```python
from build123d import *

# Parameters (mm, degrees)
BOSS_EXTRUDE1_DEPTH = 1.5
FILLET1_R           = 1.5875
SKETCH2_W           = 3
SKETCH2_H           = 6.35
BOSS_EXTRUDE2_DEPTH = 3
FILLET2_R           = 0.79375


with BuildPart() as part:
    # Sketch1 → Boss-Extrude1 (new, symmetric)
    with BuildSketch(Plane(origin=(0, 0, 0), x_dir=(1, 0, 0), z_dir=(0, 1, 0))):
        Polygon((25.4, 5.08), (9.525, 5.08), (9.525, -5.08), (25.4, -5.08), (25.4, -17.78), (6.592009247, -17.78), (0, -17.78), (-12.457990753, -17.78), (-25.4, -17.78), (-25.4, -5.08), (-9.525, -5.08), (-9.525, 5.08), (-25.4, 5.08), (-25.4, 17.78), (25.4, 17.78), align=None)
    extrude(amount=BOSS_EXTRUDE1_DEPTH, both=True)

    # Fillet1
    fillet1_edges = [part.edges().sort_by_distance(p)[0] for p in [
        (25.4, 0, -17.78),
        (25.4, 0, -5.08),
        (9.525, 0, -5.08),
        (9.525, 0, 5.08),
        (25.4, 0, 5.08),
        (25.4, 0, 17.78),
        (-25.4, 0, 17.78),
        (-25.4, 0, 5.08),
        (-9.525, 0, 5.08),
        (-9.525, 0, -5.08),
        (-25.4, 0, -5.08),
        (-25.4, 0, -17.78),
    ]]
    fillet(fillet1_edges, radius=FILLET1_R)

    # Sketch2 → Boss-Extrude2 (add)
    with BuildSketch(Plane(origin=(0, 1.5, 0), x_dir=(1, 0, 0), z_dir=(0, 1, 0))):
        with Locations((-26.9, 11.43)):
            Rectangle(SKETCH2_W, SKETCH2_H)
        with Locations((26.9, 11.43)):
            Rectangle(SKETCH2_W, SKETCH2_H)
        with Locations((26.9, -11.43)):
            Rectangle(SKETCH2_W, SKETCH2_H)
        with Locations((-26.9, -11.43)):
            Rectangle(SKETCH2_W, SKETCH2_H)
    extrude(amount=-BOSS_EXTRUDE2_DEPTH)

    # Fillet2
    fillet2_edges = [part.edges().sort_by_distance(p)[0] for p in [
        (-28.4, 0, 14.605),
        (-28.4, 0, 8.255),
        (28.4, 0, 8.255),
        (28.4, 0, 14.605),
        (28.4, 0, -14.605),
        (28.4, 0, -8.255),
        (-28.4, 0, -8.255),
        (-28.4, 0, -14.605),
    ]]
    fillet(fillet2_edges, radius=FILLET2_R)


solid = part.part
```
Source: CAD feature listing. Evaluate the final solid. Frame: model axes, mm. A direction names the side the tool comes from. Coordinates: 2 decimals unless noted, no trailing zeros. Loops run counter-clockwise (first coordinate to the right, second up) from the corner with the lowest first, then second, coordinate; pieces in that order, holes last. Notation, with made-up numbers: (39.25, 69) - (94.25, 69) arc R21 cw to (94.25, 97) - close; hole circle Ø3 at (-7.75, 70). An arc over 180 degrees is marked (long way). Answer as CSV lines item,"result".
1. Section A-A (x = 19.5). Return loops of the section in (y, z).
Established:
outline,"(-1.5, -17.78) - (1.5, -17.78) - (1.5, -5.08) - (-1.5, -5.08) - close; (-1.5, 5.08) - (1.5, 5.08) - (1.5, 17.78) - (-1.5, 17.78) - close"
2. Reachability of faces 1 (the flat face through (-27, 0, -8.255)), 2 (the flat face through (26, 0, 14.605)), 3 (the flat face through (9.525, 0, 0)), 4 (the flat face through (25.4, 0, -15)) from +Z, -Z, +X, -X, +Y, -Y: full face, straight path, thin tool, end or side. Return the list, or none.
Established:
face 1,"-X, +Y, -Y"
face 2,"+Z, +X, +Y, -Y"
face 3,"+X, +Y, -Y"
face 4,"-Z, +X, +Y, -Y"
3. Ray query, line 1 (Z direction, x = -12, y = -1.15); line 2 (Z direction, x = 10.5, y = 0.05); line 3 (X direction, y = -1.2, z = 7.5). Return the intervals inside material, ascending.
Established:
line 1,"z = -17.78 to -5.08, 5.08 to 17.78"
line 2,"z = -17.78 to -4.96, 4.96 to 17.78"
line 3,"x = -25.4 to 25.4"
4. Contact query for flat-ended pins moving along their axis: pin 1 (0.8 mm diameter, centred on y = 0.5, z = 7.5, fed in from +X); pin 2 (0.8 mm diameter, centred on y = -0.5, z = 15.5, fed in from -X); pin 3 (1 mm diameter, centred on y = 0.5, z = 3.5, fed in from -X). Output: stop coordinate, or through.
Established:
pin 1,"stops at x = 25.4"
pin 2,"stops at x = -25.4"
pin 3,"stops at x = -9.61"
5. Mould query, pull axis Z, two halves, no side actions, for faces 5 (the cylindrical face through (-24.92, -0.02, 5.53)), 6 (the flat face through (0, 0, -17.78)), 7 (the flat face through (0, -1.5, 0)). Classes: released by +Z, released by -Z, zero draft, split by the parting line, or undercut.
Established:
face 5,"undercut"
face 6,"released by -Z"
face 7,"zero draft"
